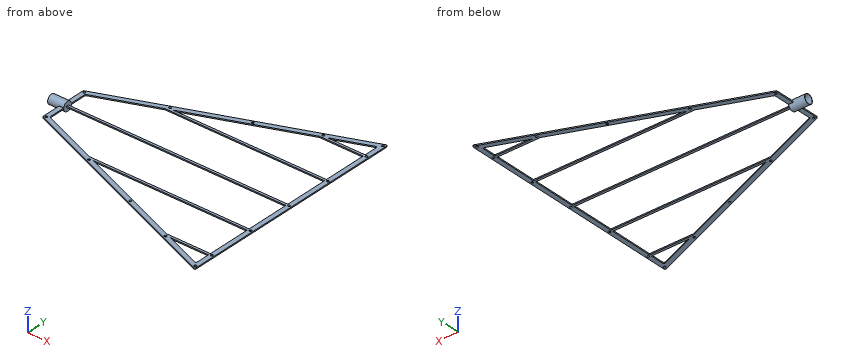
```python
from build123d import *

# Parameters (mm, degrees)
EXTRUDE_1_DEPTH     = 0.25
SKETCH_4_R          = 0.5
CUT_EXTRUDE_1_DEPTH = 0.25
FILLET_1_R          = 0.5


with BuildPart() as part:
    # 草图1 → 凸台-拉伸1 (new body, symmetric)
    with BuildSketch(Plane.XY):
        Polygon((0, -10.5), (0, 10.5), (99.442194264, 50), (99.442194264, -50), align=None)
        Polygon((2, 9.142427382), (28.075436668, 19.5), (97.442194264, 19.5), (97.442194264, 0.5), (2, 0.5), align=None, mode=Mode.SUBTRACT)
        Polygon((97.442194264, 47.053564614), (97.442194264, 40.5), (80.943438681, 40.5), align=None, mode=Mode.SUBTRACT)
        Polygon((97.442194264, -47.053564614), (80.943438681, -40.5), (97.442194264, -40.5), align=None, mode=Mode.SUBTRACT)
        Polygon((2, -9.142427382), (2, -0.5), (97.442194264, -0.5), (97.442194264, -19.5), (28.075436668, -19.5), align=None, mode=Mode.SUBTRACT)
        Polygon((30.592960573, 20.5), (97.442194264, 20.5), (97.442194264, 39.5), (78.425914776, 39.5), align=None, mode=Mode.SUBTRACT)
        Polygon((78.425914776, -39.5), (97.442194264, -39.5), (97.442194264, -20.5), (30.592960573, -20.5), align=None, mode=Mode.SUBTRACT)
    extrude(amount=EXTRUDE_1_DEPTH, both=True)

    # 草图4 → 切除-拉伸1 (cut, symmetric)
    with BuildSketch(Plane.XY):
        with Locations((1, 9.821213691)):
            Circle(SKETCH_4_R)
        with Locations((29, 20.943253065)):
            Circle(SKETCH_4_R)
        with Locations((56, 31.668076746)):
            Circle(SKETCH_4_R)
        with Locations((79, 40.80403766)):
            Circle(SKETCH_4_R)
        with Locations((98.442194264, 48.526782307)):
            Circle(SKETCH_4_R)
        with Locations((98.442194264, 40)):
            Circle(SKETCH_4_R)
        with Locations((98.442194264, 20)):
            Circle(SKETCH_4_R)
        with Locations((98.442194264, 0)):
            Circle(SKETCH_4_R)
        with Locations((98.442194264, -20)):
            Circle(SKETCH_4_R)
        with Locations((98.442194264, -40)):
            Circle(SKETCH_4_R)
        with Locations((98.442194264, -48.526782307)):
            Circle(SKETCH_4_R)
        with Locations((79, -40.80403766)):
            Circle(SKETCH_4_R)
        with Locations((56, -31.668076746)):
            Circle(SKETCH_4_R)
        with Locations((29, -20.943253065)):
            Circle(SKETCH_4_R)
        with Locations((1, -9.821213691)):
            Circle(SKETCH_4_R)
    extrude(amount=CUT_EXTRUDE_1_DEPTH, both=True, mode=Mode.SUBTRACT)

    # 草图5 → 旋转1 (revolve)
    with BuildSketch(Plane.XY):
        Polygon((2, 0), (2, 2), (-5, 2), (-5, 1.9), (0, 1.9), (0, 0), align=None)
    revolve(axis=Axis((0, 0, 0), (-1, 0, 0)))

    # 圆角1
    fillet_1_edges = [part.edges().sort_by_distance(p)[0] for p in [
        (2, 9.142427382, 0),
        (97.442194264, 47.053564614, 0),
        (97.442194264, -47.053564614, 0),
        (2, -9.142427382, 0),
        (99.442194264, 50, 0),
        (99.442194264, -50, 0),
        (0, -10.5, 0),
        (0, 10.5, 0),
    ]]
    fillet(fillet_1_edges, radius=FILLET_1_R)


solid = part.part
```
Could you check a few things on this model? Use its own coordinates, in mm. Coordinates: 2 decimals unless noted, no trailing zeros. Write each loop counter-clockwise with the first axis right and the second up, starting at its lowest first coordinate (ties: lowest second). Pieces come first, ordered by that corner, then holes. Notation, with made-up numbers: (-36.75, 72) - (5.25, 72) arc R23 ccw to (5.25, 85) - close; hole circle Ø11 at (42.25, 47). An arc over 180 degrees is marked (long way). Use a Markdown table: item, result.
Q1. Imagine slicing it at C-C (x = 43.5). List the corners of the cut face in (y, z) for me.
Geometry check:
| item | result |
|---|---|
| outline | (-27.78, -0.25) - (-25.63, -0.25) - (-25.63, 0.25) - (-27.78, 0.25) - close; (-20.5, -0.25) - (-19.5, -0.25) - (-19.5, 0.25) - (-20.5, 0.25) - close; (-0.5, -0.25) - (0.5, -0.25) - (0.5, 0.25) - (-0.5, 0.25) - close; (19.5, -0.25) - (20.5, -0.25) - (20.5, 0.25) - (19.5, 0.25) - close; (25.63, -0.25) - (27.78, -0.25) - (27.78, 0.25) - (25.63, 0.25) - close |
Q2. Imagine slicing it at A-A (y = 5). List the corners of the cut face in (x, z) for me.
Geometry check:
| item | result |
|---|---|
| outline | (0, -0.25) - (2, -0.25) - (2, 0.25) - (0, 0.25) - close; (97.44, -0.25) - (99.44, -0.25) - (99.44, 0.25) - (97.44, 0.25) - close |
Q3. Imagine slicing it at D-D (y = 42.5). List the corners of the cut face in (x, z) for me, and give its area (3 significant figures).
Geometry check:
| item | result |
|---|---|
| outline | (80.56, -0.25) - (85.98, -0.25) - (85.98, 0.25) - (80.56, 0.25) - close; (97.44, -0.25) - (99.44, -0.25) - (99.44, 0.25) - (97.44, 0.25) - close |
| area | 3.71 mm2 |
Q4. Imagine slicing it at B-B (x = 82.5). List the corners of the cut face in (y, z) for me, and give its area (3 significant figures).
Geometry check:
| item | result |
|---|---|
| outline | (-43.27, -0.25) - (-41.12, -0.25) - (-41.12, 0.25) - (-43.27, 0.25) - close; (-40.5, -0.25) - (-39.5, -0.25) - (-39.5, 0.25) - (-40.5, 0.25) - close; (-20.5, -0.25) - (-19.5, -0.25) - (-19.5, 0.25) - (-20.5, 0.25) - close; (-0.5, -0.25) - (0.5, -0.25) - (0.5, 0.25) - (-0.5, 0.25) - close; (19.5, -0.25) - (20.5, -0.25) - (20.5, 0.25) - (19.5, 0.25) - close; (39.5, -0.25) - (40.5, -0.25) - (40.5, 0.25) - (39.5, 0.25) - close; (41.12, -0.25) - (43.27, -0.25) - (43.27, 0.25) - (41.12, 0.25) - close |
| area | 4.65 mm2 |
Q5. Please list where these lines run through material, in increasing order: L1, parallel to Y at x = 29, z = -0.1; L2, parallel to X at y = -1, z = -0.7; L3, parallel to Y at x = 22, z = -0.15.
Geometry check:
| item | result |
|---|---|
| L1 | y = -22.02 to -21.44, -20.44 to -19.5, -0.5 to 0.5, 19.5 to 20.44, 21.44 to 22.02 |
| L2 | x = 0 to 2 |
| L3 | y = -19.24 to -17.09, -0.5 to 0.5, 17.09 to 19.24 |
Q6. I'm going to push flat-ended pins straight in: pin 1 Ø1.2 at (y, z) = (-0.5, -0.5) entering from +X; pin 2 Ø0.6 at (x, z) = (57.5, 0) entering from +Y; pin 3 Ø0.6 at (x, z) = (88, 0) entering from +Y; pin 4 Ø10 at (x, y) = (62, -24) entering from -Z. Where does each tip first touch, or does it pass through?
Geometry check:
| item | result |
|---|---|
| pin 1 | stops at x = 99.44 |
| pin 2 | stops at y = 33.46 |
| pin 3 | stops at y = 45.57 |
| pin 4 | stops at z = -0.25 |
